Check sheet for the drawn part. Datum: minimum x, y, z corner. Units: mm. Round coordinates to 2 decimals unless told otherwise and drop trailing zeros. Order: outer loops, then holes, each group sorted by start corner. A loop starts at its lowest first (then second) coordinate and runs counter-clockwise, first axis right, second up.
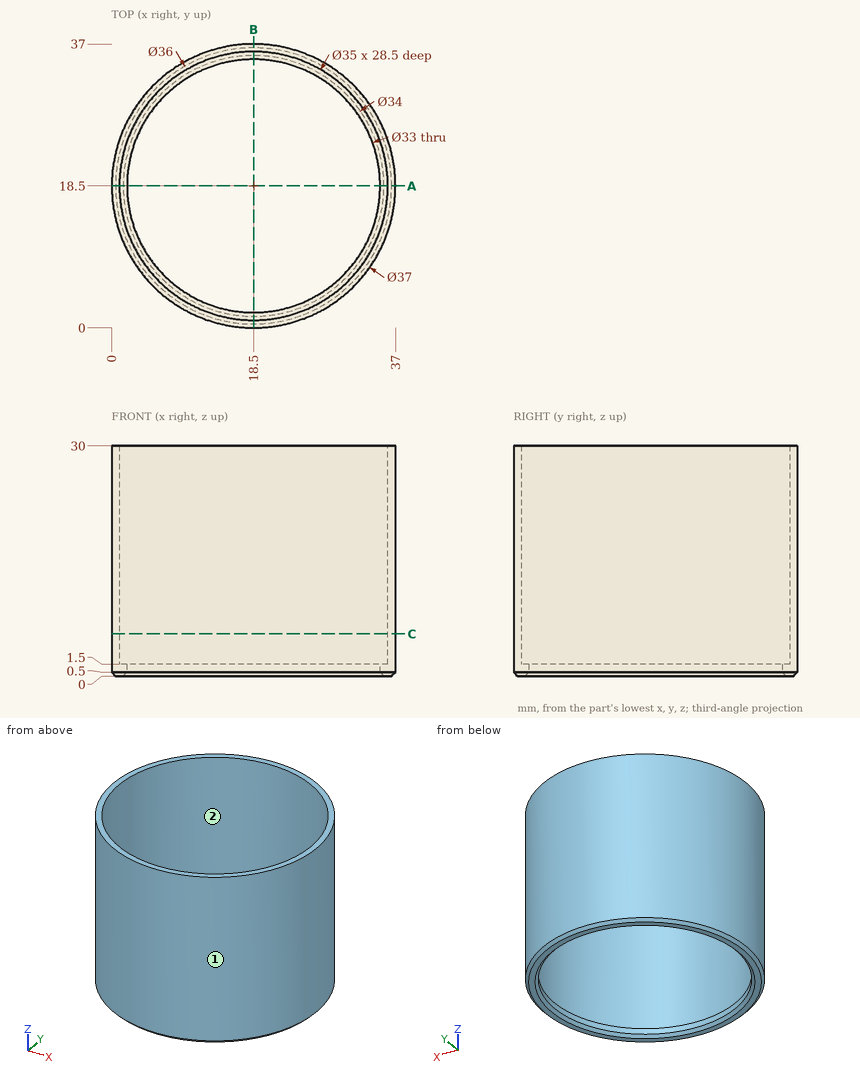
(1) Draft check along Y on the marked faces 1 and 2. Enter one of: released by +Y, released by -Y, zero draft, split by the parting line, or undercut.
Returned:
face 1: split by the parting line
face 2: undercut
(2) Sectioned sample at C-C, the plane z = 5.5. Record the cut outline in (x, y).
Returned:
outline: circle Ø37 at (18.5, 18.5); hole circle Ø35 at (18.5, 18.5)
(3) Material ranges on line 1 (Y direction, x = 18.5, z = 1.35); line 2 (Y direction, x = 18.5, z = 9); line 3 (X direction, y = 18, z = 12.5), recorded low to high.
Returned:
line 1: y = 0 to 2, 35 to 37
line 2: y = 0 to 1, 36 to 37
line 3: x = 0.01 to 1.01, 35.99 to 36.99
(4) Sectioned sample at A-A, the plane y = 18.5. Record the cut outline in (x, z).
Returned:
outline: (0, 0.5) - (0.5, 0) - (1.5, 0) - (2, 0.5) - (2, 1.5) - (1, 1.5) - (1, 30) - (0, 30) - close; (35, 0.5) - (35.5, 0) - (36.5, 0) - (37, 0.5) - (37, 30) - (36, 30) - (36, 1.5) - (35, 1.5) - close
(5) Depth check by flat-ended pin: P1, Ø3, axis at y = 20, z = 18.5, coming from the -X side; P2, Ø3, axis at x = 14.5, z = 25.5, coming from the -Y side; P3, Ø1, axis at x = 13, z = 4.5, coming from the +Y side; P4, Ø12, axis at y = 33, z = 23.5, coming from the -X side. Enter the tip coordinate at first touch or a pass-through.
Returned:
P1: stops at x = 0
P2: stops at y = 0.17
P3: stops at y = 36.31
P4: stops at x = 2.07
